from build123d import *

# Parameters (mm, degrees)
F0_W     = 10
F0_H     = 10
F0_R     = 1.65
F1_DEPTH = 7
F0_R_2   = 4.65
F2_DEPTH = 2
F3_SIZE  = 2


with BuildPart() as f1:
    # F0 (on Top) → F1 (new body)
    with BuildSketch(Plane.XY):
        with Locations((25, -41.75)):
            Rectangle(F0_W, F0_H)
        with Locations((25, -41.75)):
            Circle(F0_R, mode=Mode.SUBTRACT)
    extrude(amount=F1_DEPTH)



with BuildPart() as f1b:
    # F0 (on Top) → F1, piece 2 (new body)
    with BuildSketch(Plane.XY):
        with Locations((25, -8.25)):
            Rectangle(F0_W, F0_H)
        with Locations((25, -8.25)):
            Circle(F0_R, mode=Mode.SUBTRACT)
    extrude(amount=F1_DEPTH)


with BuildPart() as f1_1:
    add(f1.part)

    add(f1b.part)  # F2 merges F1b
    # F0 (on Top) → F2 (join)
    with BuildSketch(Plane.XY):
        with BuildLine():
            Line((45, 0), (5, 0))
            ThreePointArc((5, 0), (1.4644660941, -1.4644660941), (0, -5))
            Line((0, -5), (0, -45))
            ThreePointArc((0, -45), (1.4644660941, -48.5355339059), (5, -50))
            Line((5, -50), (45, -50))
            ThreePointArc((45, -50), (48.5355339059, -48.5355339059), (50, -45))
            Line((50, -45), (50, -5))
            ThreePointArc((50, -5), (48.5355339059, -1.4644660941), (45, 0))
        make_face()
        with Locations((7.0710678119, -42.9289321881)):
            Circle(F0_R_2, mode=Mode.SUBTRACT)
        with Locations((25, -41.75)):
            Rectangle(F0_W, F0_H, mode=Mode.SUBTRACT)
        with Locations((42.9289321881, -42.9289321881)):
            Circle(F0_R_2, mode=Mode.SUBTRACT)
        with Locations((7.0710678119, -7.0710678119)):
            Circle(F0_R_2, mode=Mode.SUBTRACT)
        with Locations((25, -8.25)):
            Rectangle(F0_W, F0_H, mode=Mode.SUBTRACT)
        with Locations((42.9289321881, -7.0710678119)):
            Circle(F0_R_2, mode=Mode.SUBTRACT)
    extrude(amount=F2_DEPTH)

    # F3
    f3_edges = [f1_1.edges().sort_by_distance(p)[0] for p in [
        (25, -46.75, 2),
        (30, -8.25, 2),
        (30, -41.75, 2),
        (25, -13.25, 2),
        (25, -3.25, 2),
        (25, -36.75, 2),
        (20, -8.25, 2),
        (20, -41.75, 2),
    ]]
    chamfer(f3_edges, length=F3_SIZE)


solid = f1_1.part
Work out the finished part from the listing and answer in its coordinate system (mm). A direction names the side the tool comes from. Coordinates: 2 decimals unless noted, no trailing zeros. Loops run counter-clockwise (first coordinate to the right, second up) from the corner with the lowest first, then second, coordinate; pieces in that order, holes last. Notation, with made-up numbers: M -16.5,76 L 16.5,76 A13 ccw 16.5,96 Z; hole C 36.25,15 d10. An arc over 180 degrees is marked long. Answer in a Markdown table with one row per item. Add a question column.
1. Flat-ended cylindrical pins translate along their axes: P1, Ø0.9, axis at y = -44, z = 5, coming from the +X side; P2, Ø2, axis at x = 16.5, y = -31, coming from the +Z side; P3, Ø3.5, axis at y = -44, z = 5.5, coming from the -X side. Find the tip coordinate at first contact, or state that the pin passes through.
2. Consider L1, parallel to X at y = -7, z = 1; L2, parallel to Y at x = 25, z = 3; L3, parallel to Y at x = 27, z = 5.5. Determine where each line is inside the solid, lowest interval first.
3. Find section D-D, the plane y = -8.25. Write down the section's boundary in (x, z), then the cut area to 3 significant figures.
4. A tool of negligible diameter and unlimited length cuts with its end or side. For faces 5 (the flat face through (25, -3.25, 5)), 6 (the flat face through (25, -25, 2)), 7 (the flat face through (30, -42, 5)), 8 (the flat face through (20, -42, 5)), from which of +Z, -Z, +X, -X, +Y, -Y can it reach the whole face along a straight path? Write none if from no direction.
5. Find section A-A, the plane z = 4.75. Write down the section's boundary in (x, y), then the cut area to 3 significant figures.
6. The mould has two halves that part along Y. Classify faces 1 (the cylindrical face through (3.38, -9.9, 0.99)), 2 (the flat face through (25, -25, 0)), 3 (the flat face through (25, 0, 1)), 4 (the flat face through (24.9, -14.24, 3.01)): pulls with the +Y half, pulls with the -Y half, needs draft (parallel to the pull), parting line crosses it, or undercut.
7. Find section B-B, the plane x = 25. Write down the section's boundary in (y, z), then the cut area to 3 significant figures.
8. Find section C-C, the plane y = -37.5. Write down the section's boundary in (x, z).
Reported:
| question | item | result |
|---|---|---|
| 1 | P1 | stops at x = 30 |
| 1 | P2 | stops at z = 2 |
| 1 | P3 | stops at x = 19.75 |
| 2 | L1 | x = 0 to 2.42, 11.72 to 23.92, 26.08 to 38.28, 47.58 to 50 |
| 2 | L2 | y = -47.75 to -43.4, -40.1 to -35.75, -14.25 to -9.9, -6.6 to -2.25 |
| 2 | L3 | y = -46.75 to -36.75, -13.25 to -3.25 |
| 3 | outline | M 0,0 L 2.57,0 L 2.57,2 L 0,2 Z; M 11.57,0 L 23.35,0 L 23.35,7 L 20,7 L 20,4 L 18,2 L 11.57,2 Z; M 26.65,0 L 38.43,0 L 38.43,2 L 32,2 L 30,4 L 30,7 L 26.65,7 Z; M 47.43,0 L 50,0 L 50,2 L 47.43,2 Z |
| 3 | area | 94.9 mm^2 |
| 4 | face 5 | +Z, +X, -X, +Y |
| 4 | face 6 | +Z |
| 4 | face 7 | +Z, +X, +Y, -Y |
| 4 | face 8 | +Z, -X, +Y, -Y |
| 5 | outline | M 20,-46.75 L 30,-46.75 L 30,-36.75 L 20,-36.75 Z; M 20,-13.25 L 30,-13.25 L 30,-3.25 L 20,-3.25 Z; hole C 25,-41.75 d3.3; hole C 25,-8.25 d3.3 |
| 5 | area | 183 mm^2 |
| 6 | face 1 | undercut |
| 6 | face 2 | needs draft |
| 6 | face 3 | pulls with the +Y half |
| 6 | face 4 | undercut |
| 7 | outline | M -50,0 L -43.4,0 L -43.4,7 L -46.75,7 L -46.75,4 L -48.75,2 L -50,2 Z; M -40.1,0 L -9.9,0 L -9.9,7 L -13.25,7 L -13.25,4 L -15.25,2 L -34.75,2 L -36.75,4 L -36.75,7 L -40.1,7 Z; M -6.6,0 L 0,0 L 0,2 L -1.25,2 L -3.25,4 L -3.25,7 L -6.6,7 Z |
| 7 | area | 162 mm^2 |
| 8 | outline | M 0,0 L 50,0 L 50,2 L 32,2 L 30,4 L 30,7 L 20,7 L 20,4 L 18,2 L 0,2 Z |
